Check sheet for the modelled part. Datum: model origin and axes. Units: mm. A direction names the side the tool comes from. Round coordinates to 2 decimals unless told otherwise and drop trailing zeros. Order: outer loops, then holes, each group sorted by start corner. A loop starts at its lowest first (then second) coordinate and runs counter-clockwise, first axis right, second up.
(1) Mould release check, pull along Y, two halves, no side actions. Record for faces 4 (the conical face through (0.07, 45.36, 0.33)), 5 (the cylindrical face through (3.32, -14.9, -3.04)), 6 (the conical face through (-1.903, 26.625, -3.66)), 7 (the flat face through (0, -44.5, 0)): released by +Y, released by -Y, zero draft, split by the parting line, or undercut.
(2) Sectioned sample at A-A, the plane y = -37.5. Enter the section's corners in (x, z).
(3) Depth check by flat-ended pin: pin 1 (1.5 mm diameter, centred on x = -1, y = -3, fed in from -Z); pin 2 (3 mm diameter, centred on y = -41, z = -1, fed in from +X); pin 3 (1 mm diameter, centred on x = -4.5, z = -4, fed in from -Y). Enter the tip coordinate at first touch or a pass-through.
(4) Thickness scan on probe 1 along Y at (x, z) = (-1.5, 2.75); probe 2 along Y at (x, z) = (-1, -4.25); probe 3 along Z at (x, y) = (0, 25.5). Record the ranges inside material, lowest first.
(5) Tool access check on faces 1 (the flat face through (-3.55, -40, 0)), 2 (the flat face through (0, -40, 3.55)), 3 (the cylindrical face through (0.867, 15.346, 3.905)). Record the directions out of +Z, -Z, +X, -X, +Y, -Y that give a thin tool (end or side, any length) a straight path to the whole face; none if there is none.
(6) Sectioned sample at B-B, the plane y = -15. Enter the section's corners in (x, z).
(7) Sectioned sample at C-C, the plane y = 24.5. Enter the section's corners in (x, z).
Autodesk Inventor part; units mm, degrees
ref_plane "YZ Plane" through (0, 0, 0) normal (1, 0, 0) x (0, 1, 0)
ref_plane "XZ Plane" through (0, 0, 0) normal (0, 1, 0) x (-1, 0, 0)
ref_plane "XY Plane" through (0, 0, 0) normal (0, 0, 1) x (1, 0, 0)
sketch "Sketch1" plane through (0, 0, 0) normal (0, 0, 1) x (1, 0, 0)
  line L0 (-7.2, 0) -> (1.2, 0) construction
  line L1 (0, -62.54) -> (0, 63.74)
  line L2 (0, 45.7) -> (-1.2, 44.5)
  line L3 (-1.2, 44.5) -> (-5.65, 44.5)
  line L4 (-5.65, 44.5) -> (-6, 40.5)
  line L5 (-6, 40.5) -> (-6, 28.5)
  line L6 (-4, 26.5) -> (-4, 4.5)
  line L7 (-4, 4.5) -> (-4.5, 4.5)
  line L8 (-4.5, 4.5) -> (-4.5, -44.5)
  line L9 (-4.5, -44.5) -> (0, -44.5)
  line L10 (-6, 28.5) -> (-4, 26.5)
  point P0 (0, 0)
  dimension "tdz" = 12
  dimension "d1" = 45
  dimension "d2" = 5
  dimension "thl" = 16
  dimension "lu" = 40
  dimension "oal" = 89
  dimension "d6" = 1.2
  dimension "d7" = 4
  dimension "dconms" = 9
  dimension "d9" = 8
  dimension "d11" = 45
revolve "Revolution1" add sketch "Sketch1" angle 360 about axis through (0, -10, 0) along (0, 1, 0)
sketch "Sketch2" plane through (0, -44.5, 0) normal (0, -1, 0) x (1, 0, 0)
  circle A0 centre (0, 0) radius 4.5 construction
  line L0 (3.55, 3.55) -> (3.55, -3.55)
  line L1 (3.55, -3.55) -> (-3.55, -3.55)
  line L2 (-3.55, -3.55) -> (-3.55, 3.55)
  line L3 (-3.55, 3.55) -> (3.55, 3.55)
  circle A1 centre (0, 0) radius 6
  dimension "d12" = 7.1
extrude "Extrusion1" cut sketch "Sketch2" against normal blind 10
equation "\"d6\" = 0.1 * tdz"
equation "\"d7\" = 0.25 * thl"
properties part number "Tap"
Derived:
1. face 4: released by +Y
1. face 5: zero draft
1. face 6: undercut
1. face 7: released by -Y
2. outline: (-3.55, -2.77) arc R4.5 ccw to (-2.77, -3.55) - (2.77, -3.55) arc R4.5 ccw to (3.55, -2.77) - (3.55, 2.77) arc R4.5 ccw to (2.77, 3.55) - (-2.77, 3.55) arc R4.5 ccw to (-3.55, 2.77) - close
3. pin 1: stops at z = -4.49
3. pin 2: stops at x = 3.55
3. pin 3: stops at y = 28.02
4. probe 1: y = -44.5 to 44.5
4. probe 2: y = -34.5 to 4.5, 26.87 to 44.5
4. probe 3: z = -4 to 4
5. face 1: +Z, -Z, -X, -Y
5. face 2: +Z, +X, -X, -Y
5. face 3: none
6. outline: circle Ø9 at (0, 0)
7. outline: circle Ø8 at (0, 0)
